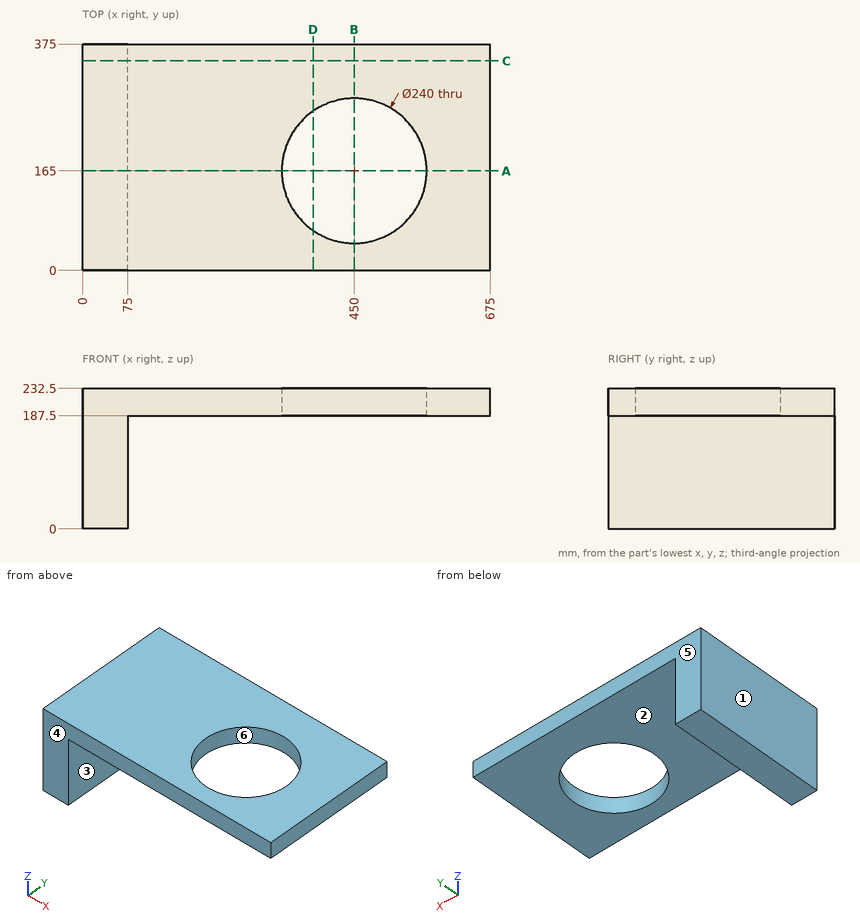
Can you work these out from the drawing? Everything is in mm from the part's minimum corner. A direction names the side the tool comes from. Coordinates: 2 decimals unless noted, no trailing zeros. Loops run counter-clockwise (first coordinate to the right, second up) from the corner with the lowest first, then second, coordinate; pieces in that order, holes last.
1) Which directions (+Z, -Z, +X, -X, +Y, -Y) give clear straight access to the entire face, cutting with the end or side of a thin tool? Please do the marked faces 1 and 2.
Reported:
face 1: +Z, -Z, -X, +Y, -Y
face 2: -Z, +X, +Y, -Y
2) Imagine slicing it at D-D (x = 382). List the corners of the cut face in (y, z) for me, and give its area (3 significant figures).
Reported:
outline: (0, 187.5) - (66.13, 187.5) - (66.13, 232.5) - (0, 232.5) - close; (263.87, 187.5) - (375, 187.5) - (375, 232.5) - (263.87, 232.5) - close
area: 7,980 mm2
3) Please list where these lines run through material, in increasing order: line 1 along Y through (x, z) = (450, 204); line 2 along Z through (x, y) = (256.5, 289.5); line 3 along X through (y, z) = (248.5, 177).
Reported:
line 1: y = 0 to 45, 285 to 375
line 2: z = 187.5 to 232.5
line 3: x = 0 to 75
4) Imagine slicing it at B-B (x = 450). List the corners of the cut face in (y, z) for me, and give its area (4 significant figures).
Reported:
outline: (0, 187.5) - (45, 187.5) - (45, 232.5) - (0, 232.5) - close; (285, 187.5) - (375, 187.5) - (375, 232.5) - (285, 232.5) - close
area: 6,075 mm2
5) Will these pins go through, and if not, where does the flat tip stop? pin 1 Ø10 at (x, y) = (149.5, 105) entering from -Z; pin 2 Ø8 at (y, z) = (308.5, 34) entering from +X; pin 3 Ø1.5 at (y, z) = (233, 79) entering from -X.
Reported:
pin 1: stops at z = 187.5
pin 2: stops at x = 75
pin 3: stops at x = 0
6) Imagine slicing it at C-C (y = 347). List the corners of the cut face in (x, z) for me, and give its area (3 significant figures).
Reported:
outline: (0, 0) - (75, 0) - (75, 187.5) - (675, 187.5) - (675, 232.5) - (0, 232.5) - close
area: 44,400 mm2
7) Imagine slicing it at A-A (y = 165). List the corners of the cut face in (x, z) for me, and give its area (3 significant figures).
Reported:
outline: (0, 0) - (75, 0) - (75, 187.5) - (330, 187.5) - (330, 232.5) - (0, 232.5) - close; (570, 187.5) - (675, 187.5) - (675, 232.5) - (570, 232.5) - close
area: 33,600 mm2
8) Thinking about a two-plate mould opening in Y: for the marked faces 3, 4, 5 and 6, which applies, released by +Y, released by -Y, zero draft, split by the parting line, or undercut?
Reported:
face 3: zero draft
face 4: released by -Y
face 5: released by +Y
face 6: undercut
